Autodesk Inventor part; units mm, degrees
ref_plane "YZ Plane" through (0, 0, 0) normal (1, 0, 0) x (0, 1, 0)
ref_plane "XZ Plane" through (0, 0, 0) normal (0, 1, 0) x (-1, 0, 0)
ref_plane "XY Plane" through (0, 0, 0) normal (0, 0, 1) x (1, 0, 0)
sketch "Esboço1" plane through (0, 0, 0) normal (0, 0, 1) x (1, 0, 0)
  line L0 (0, 0) -> (50, 0)
  line L1 (50, 0) -> (50, 70)
  line L2 (50, 70) -> (40, 70)
  line L3 (40, 70) -> (40, 10)
  line L4 (40, 10) -> (10, 10)
  line L5 (10, 10) -> (10, 50)
  line L6 (10, 50) -> (0, 50)
  line L7 (0, 50) -> (0, 0)
  dimension "d0" = 10
  dimension "d1" = 10
  dimension "d2" = 10
  dimension "d3" = 50
  dimension "d4" = 50
  dimension "d5" = 70
extrude "Extrusão1" add sketch "Esboço1" along normal blind 1020
sketch "Esboço2" plane through (0, 0, 1020) normal (0, 0, 1) x (1, 0, 0)
  line L0 (0, 0) -> (50, 0)
  line L1 (0, 0) -> (50, 0)
  line L2 (50, 0) -> (50, 50)
  line L3 (50, 50) -> (0, 50)
  line L4 (10, 10) -> (10, 50)
  line L5 (0, 50) -> (0, 0)
  line L6 (0, 50) -> (0, 0)
extrude "Extrusão2" add sketch "Esboço2" against normal blind 10
sketch "Esboço3" plane through (0, 0, 0) normal (0, 0, -1) x (-1, 0, 0)
  line L0 (0, 0) -> (-50, 0)
  line L1 (-40, 50) -> (0, 50)
  line L2 (-50, 0) -> (0, 0)
  line L3 (0, 0) -> (0, 50)
  line L4 (0, 50) -> (-50, 50)
  line L5 (-50, 50) -> (-50, 0)
extrude "Extrusão3" add sketch "Esboço3" against normal blind 10
properties part number "calha"
For this review, take the finished solid that the model builds, in its own axes (mm). A direction names the side the tool comes from. Coordinates: 2 decimals unless noted, no trailing zeros. Write each loop counter-clockwise with the first axis right and the second up, starting at its lowest first coordinate (ties: lowest second). Pieces come first, ordered by that corner, then holes.
(1) Add section A-A on y = 20.5. Give the boundary of the cut face in (x, z), then the cut area to 3 significant figures.
(2) Add section C-C on z = 931. Give the boundary of the cut face in (x, y), then the cut area to 3 significant figures.
(3) The part is to be moulded in two halves that separate along X. For faces 1 (the face through (25, 28, 0)), 2 (the face through (0, 25, 503)), 3 (the face through (40, 40, 503)), say which applies: +X half, -X half, draft (parallel to the pull), parting line (faces both ways), or undercut.
(4) For pin 1 Ø15 at (x, z) = (22, 302.5) entering from +Y; pin 2 Ø10 at (x, y) = (8, 15) entering from -Z; pin 3 Ø1.5 at (y, z) = (62, 583) entering from -X; pin 4 Ø12 at (x, z) = (14.5, 492) entering from +Y, all flat-tipped, find the tip position at first contact; note any pin that passes through.
(5) Add section B-B on x = 17.5. Give the boundary of the cut face in (y, z), then the cut area to 3 significant figures.
(6) Wall thickness on probe 1 along Z at (x, y) = (27.5, 17); probe 2 along X at (y, z) = (11, 632.5); probe 3 along Y at (x, z) = (14.5, 567.5): over which ranges is each line inside the solid? List them lowest first.
(7) Tool access review of faces 4 (the face through (25, 30, 10)), 5 (the face through (7, 50, 508)), 6 (the face through (25, 0, 503)): name each direction out of +Z, -Z, +X, -X, +Y, -Y from which nothing blocks a thin tool from reaching the whole face with its end or side.
Answer sheet:
1. outline: (0, 0) - (50, 0) - (50, 1020) - (0, 1020) - close; hole (10, 10) - (40, 10) - (40, 1010) - (10, 1010) - close
1. area: 21,000 mm2
2. outline: (0, 0) - (50, 0) - (50, 70) - (40, 70) - (40, 10) - (10, 10) - (10, 50) - (0, 50) - close
2. area: 1,500 mm2
3. face 1: draft
3. face 2: -X half
3. face 3: undercut
4. pin 1: stops at y = 10
4. pin 2: stops at z = 0
4. pin 3: stops at x = 40
4. pin 4: stops at y = 50
5. outline: (0, 0) - (50, 0) - (50, 10) - (10, 10) - (10, 1010) - (50, 1010) - (50, 1020) - (0, 1020) - close
5. area: 11,000 mm2
6. probe 1: z = 0 to 10, 1010 to 1020
6. probe 2: x = 0 to 10, 40 to 50
6. probe 3: y = 0 to 10
7. face 4: +Y
7. face 5: +Z, -Z, -X, +Y
7. face 6: +Z, -Z, +X, -X, -Y
